Check sheet for the drawn part. Datum: minimum x, y, z corner. Units: mm. A direction names the side the tool comes from. Round coordinates to 2 decimals unless told otherwise and drop trailing zeros. Order: outer loops, then holes, each group sorted by start corner. A loop starts at its lowest first (then second) coordinate and runs counter-clockwise, first axis right, second up. Notation, with made-up numbers: M 14,49.5 L 26,49.5 A19 cw 26,85.5 Z; hole C 42,-18 d9. An arc over 180 degrees is marked long. Use one line per item in the form item = value. Start each with the question number.
Item 1: Go/stop test with flat-tipped pins: pin 1 Ø3 at (y, z) = (22, 11) entering from +X; pin 2 Ø4 at (y, z) = (47, 37.5) entering from +X; pin 3 Ø4 at (x, y) = (35, 6) entering from +Z; pin 4 Ø5.5 at (x, y) = (63.5, 40) entering from +Z. Record where each tip stops, or that it passes through.
Item 2: Cross-section at C-C on y = 10.5. Enter the section's corners in (x, z), then the cut area to 3 significant figures.
Item 3: Cross-section at A-A on y = 25.4. Enter the section's corners in (x, z), then the cut area to 3 significant figures.
Item 4: Cross-section at B-B on x = 37. Enter the section's corners in (y, z).
Item 5: Tool access check on the marked faces 1, 2 and 3. Record the directions out of +Z, -Z, +X, -X, +Y, -Y that give a thin tool (end or side, any length) a straight path to the whole face; none if there is none.
Item 6: Cross-section at D-D on x = 61. Enter the section's corners in (y, z), then the cut area to 3 significant figures.
Item 7: Thickness scan on probe 1 along Z at (x, y) = (48, 25); probe 2 along Y at (x, z) = (19.5, 12.7); probe 3 along Z at (x, y) = (25, 25.4). Record the ranges inside material, lowest first. Write a range as [from, to].
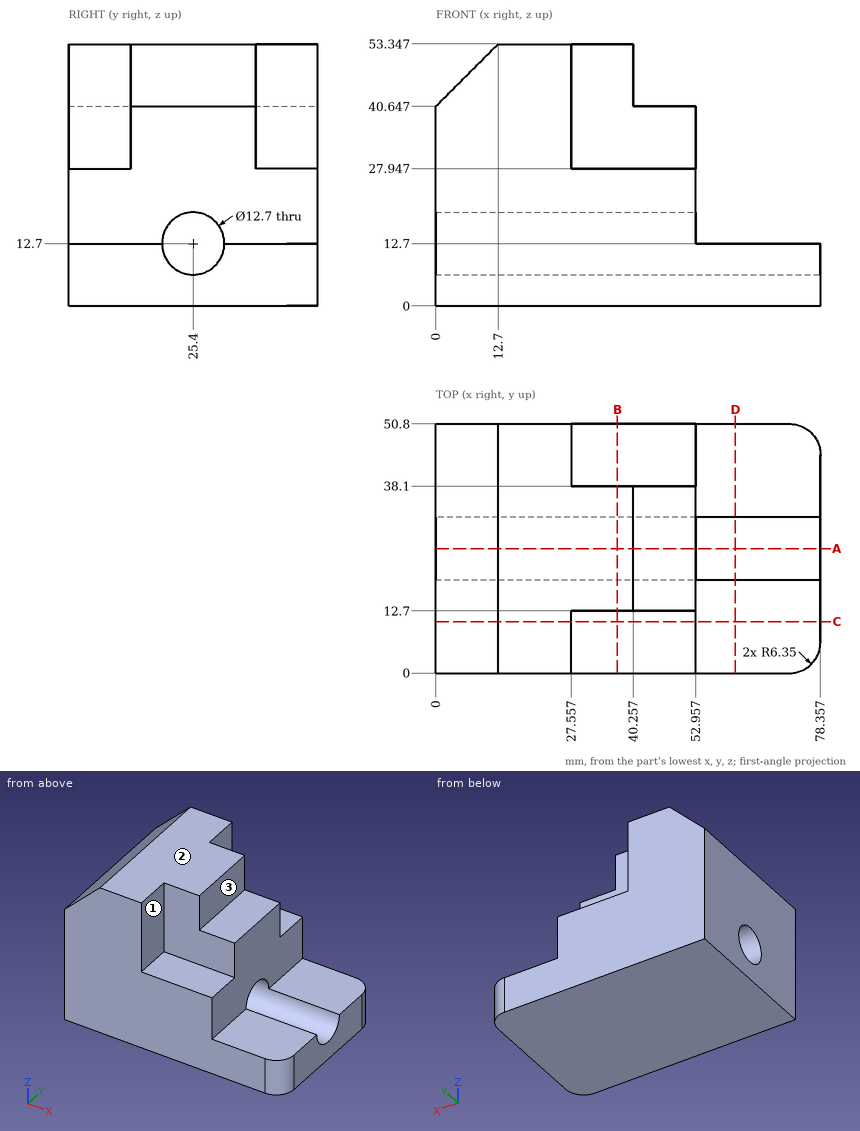
Output values:
q1.pin_1 = through
q1.pin_2 = 27.56
q1.pin_3 = 27.95
q1.pin_4 = 12.7
q2.outline = M 0,0 L 78.36,0 L 78.36,12.7 L 52.96,12.7 L 52.96,27.95 L 27.56,27.95 L 27.56,53.35 L 12.7,53.35 L 0,40.65 Z
q2.area = 2,420 mm2
q3.outline = M 0,0 L 78.36,0 L 78.36,6.35 L 0,6.35 Z; M 0,19.05 L 52.96,19.05 L 52.96,40.65 L 40.26,40.65 L 40.26,53.35 L 12.7,53.35 L 0,40.65 Z
q3.area = 2,070 mm2
q4.outline = M 0,0 L 50.8,0 L 50.8,27.95 L 38.1,27.95 L 38.1,53.35 L 12.7,53.35 L 12.7,27.95 L 0,27.95 Z; hole C 25.4,12.7 d12.7
q5.face_1 = +Z, +X, -Y
q5.face_2 = +Z, +X, -X, +Y, -Y
q5.face_3 = +Z, +X, +Y, -Y
q6.outline = M 0,0 L 50.8,0 L 50.8,12.7 L 31.75,12.7 A6.35 cw 19.05,12.7 L 0,12.7 Z
q6.area = 582 mm2
q7.probe_1 = [0, 6.36], [19.04, 40.65]
q7.probe_2 = [0, 19.05], [31.75, 50.8]
q7.probe_3 = [0, 6.35], [19.05, 53.35]
